Read the model definition and answer for the solid it produces. Units are mm, in the model's axes. Round coordinates to 2 decimals unless told otherwise and drop trailing zeros. Order: outer loops, then holes, each group sorted by start corner. A loop starts at its lowest first (then second) coordinate and runs counter-clockwise, first axis right, second up. Notation, with made-up numbers: M -2.75,-35 L 44.25,-35 A32 cw 44.25,-4 Z; hole C 30.25,17.5 d2. An arc over 180 degrees is marked long. Answer as CSV lines item,"result".
```python
from build123d import *

# Parameters (mm, degrees)
CROQUIS1_W            = 40
CROQUIS1_H            = 40
CROQUIS1_W_2          = 36
CROQUIS1_H_2          = 36
EXTRUIR_L_MINA1_DEPTH = 1060
CROQUIS2_R            = 10
EXTRUIR1_DEPTH        = 10


with BuildPart() as part:
    # Croquis1 → Extruir-Lámina1 (new body)
    with BuildSketch(Plane.XY):
        Rectangle(CROQUIS1_W, CROQUIS1_H)
        Rectangle(CROQUIS1_W_2, CROQUIS1_H_2, mode=Mode.SUBTRACT)
    extrude(amount=EXTRUIR_L_MINA1_DEPTH)

    # Croquis2 → Extruir1 (cut)
    with BuildSketch(Plane(origin=(20, 0, 0), x_dir=(0, 0, -1), z_dir=(1, 0, 0))):
        with Locations((-530, 0)):
            Circle(CROQUIS2_R)
        with Locations((-310, 0)):
            Circle(CROQUIS2_R)
        with Locations((-90, 0)):
            Circle(CROQUIS2_R)
        with Locations((-750, 0)):
            Circle(CROQUIS2_R)
        with Locations((-970, 0)):
            Circle(CROQUIS2_R)
    extrude(amount=-EXTRUIR1_DEPTH, mode=Mode.SUBTRACT)


solid = part.part
```
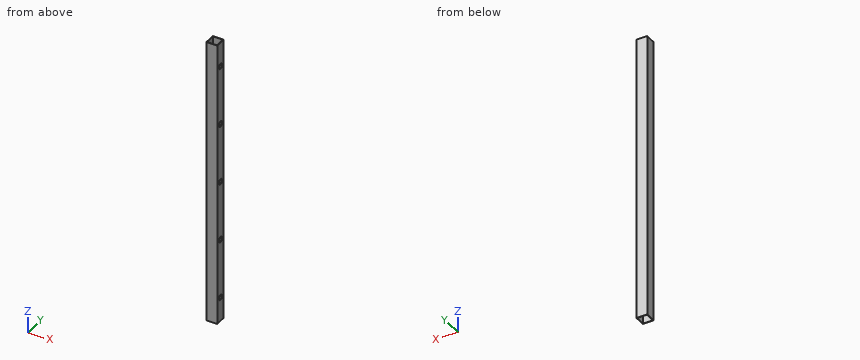
Item 1: A flat-ended cylindrical pin translates along its axis: pin 1 (16 mm diameter, centred on y = 0, z = 750, fed in from +X). Find the tip coordinate at first contact, or state that the pin passes through.
Ans:
pin 1,"x = -18"
Item 2: A cutting plane is placed at C-C, the plane z = 589. Determine the outline of the cut face in (x, y), and give its area (3 significant figures).
Ans:
outline,"M -20,-20 L 20,-20 L 20,20 L -20,20 Z; hole M -18,-18 L 18,-18 L 18,18 L -18,18 Z"
area,"304 mm2"
Item 3: A cutting plane is placed at B-B, the plane x = 9. Determine the outline of the cut face in (y, z).
Ans:
outline,"M -20,0 L -18,0 L -18,1060 L -20,1060 Z; M 18,0 L 20,0 L 20,1060 L 18,1060 Z"
Item 4: Find the intervals of material crossed by probe 1 along Y at (x, z) = (7, 992.5); probe 2 along Y at (x, z) = (19.1, 970), in increasing order. Write a range as [from, to].
Ans:
probe 1,"[-20, -18], [18, 20]"
probe 2,"[-20, -10], [10, 20]"
Item 5: A cutting plane is placed at A-A, the plane y = 0. Determine the outline of the cut face in (x, z), and give its area (3 significant figures).
Ans:
outline,"M -20,0 L -18,0 L -18,1060 L -20,1060 Z; M 18,0 L 20,0 L 20,80 L 18,80 Z; M 18,100 L 20,100 L 20,300 L 18,300 Z; M 18,320 L 20,320 L 20,520 L 18,520 Z; M 18,540 L 20,540 L 20,740 L 18,740 Z; M 18,760 L 20,760 L 20,960 L 18,960 Z; M 18,980 L 20,980 L 20,1060 L 18,1060 Z"
area,"4,040 mm2"
